Can you work these out from the model? Positions are in its coordinate system, mm. A direction names the side the tool comes from. Round coordinates to 2 decimals unless told otherwise and drop trailing zeros. Loops run counter-clockwise (first coordinate to the right, second up) from the corner with the lowest first, then second, coordinate; pieces in that order, holes last. Notation, with made-up numbers: (29.5, 76) -> (54.5, 76) arc R30 cw to (54.5, 101) -> close; hole circle Ø8 at (-32, 87.5). An arc over 180 degrees is marked (long way). Answer as a JSON object with one key per item and string values.
```python
from build123d import *

# Parameters (mm, degrees)
F0_W     = 76.6198411584
F0_H     = 75.8787617087
F1_DEPTH = 76.2
F2_W     = 13.9969550073
F2_H     = 13.1089836359
F3_DEPTH = 12.57318
F4_W     = 16.4612643421
F4_H     = 14.4383208826
F5_DEPTH = 12.45271


with BuildPart() as f1:
    # F0 (on Front) → F1 (new body)
    with BuildSketch(Plane.XZ):
        with Locations((38.3099205792, 37.9393808544)):
            Rectangle(F0_W, F0_H)
    extrude(amount=F1_DEPTH)

    # F2 (on face) → F3 (cut)
    with BuildSketch(Plane.XZ.offset(76.2)):
        with Locations((6.9984775037, 6.554491818)):
            Rectangle(F2_W, F2_H)
    extrude(amount=-F3_DEPTH, mode=Mode.SUBTRACT)

    # F4 (on Front) → F5 (cut)
    with BuildSketch(Plane.XZ):
        with Locations((68.0551026016, 7.2191604413)):
            Rectangle(F4_W, F4_H)
    extrude(amount=F5_DEPTH, mode=Mode.SUBTRACT)


solid = f1.part
```
Q1. I want a section at B-B, the plane y = -69.5. Write out the boundary of the cut face in (x, z).
Determined:
{"outline": "(0, 13.11) -> (14, 13.11) -> (14, 0) -> (76.62, 0) -> (76.62, 75.88) -> (0, 75.88) -> close"}
Q2. I want a section at A-A, the plane z = 7. Write out the boundary of the cut face in (x, y).
Determined:
{"outline": "(0, -63.63) -> (14, -63.63) -> (14, -76.2) -> (76.62, -76.2) -> (76.62, 0) -> (76.29, 0) -> (76.29, -12.45) -> (59.82, -12.45) -> (59.82, 0) -> (0, 0) -> close"}
Q3. I want a section at C-C, the plane x = 6. Write out the boundary of the cut face in (y, z), then the cut area to 3 significant figures.
Determined:
{"outline": "(-76.2, 13.11) -> (-63.63, 13.11) -> (-63.63, 0) -> (0, 0) -> (0, 75.88) -> (-76.2, 75.88) -> close", "area": "5,620 mm²"}
Q4. We'd pull the mould along X, two halves only. Please class faces 4 (the flat face through (0, -38, 37)), 5 (the flat face through (76.62, -38, 37)), 6 (the flat face through (7, -70, 13.109)), 7 (the flat face through (59.824, -6, 7)): pulls with the +X half, pulls with the -X half, needs draft (parallel to the pull), parting line crosses it, or undercut.
Determined:
{"face 4": "pulls with the -X half", "face 5": "pulls with the +X half", "face 6": "needs draft", "face 7": "undercut"}
Q5. I'm going to push flat-ended pins straight in: pin 1 (2 mm diameter, centred on x = 65, z = 11, fed in from +Y); pin 2 (6 mm diameter, centred on x = 67.5, y = -3, fed in from -Z); pin 3 (4 mm diameter, centred on x = 4, y = -68, fed in from -Z). Where does each tip first touch, or does it pass through?
Determined:
{"pin 1": "y = -12.45", "pin 2": "z = 14.44", "pin 3": "z = 13.11"}
Q6. If I drill on L1, parallel to Y at x = 72, z = 6.5, over which ranges is the centre line in solid material (lowest first)? Write a range as [from, to].
Determined:
{"L1": "[-76.2, -12.45]"}
Q7. On a 3-axis mill with a long thin cutter (end or side, diameter ignored), from which of +Z, -Z, +X, -X, +Y, -Y can I reach the whole of each face in a straight line? I mean faces 1 (the flat face through (76.286, -6, 7)), 2 (the flat face through (7, -63.627, 7)), 3 (the flat face through (38, -38, 75.879)). Say none if no direction works.
Determined:
{"face 1": "-Z, +Y", "face 2": "-Z, -X, -Y", "face 3": "+Z, +X, -X, +Y, -Y"}
